from build123d import *

# Parameters (mm, degrees)
SKETCH1_W                                       = 751.2004
SKETCH1_H                                       = 516
SKETCH1_R                                       = 42.5
BOSS_EXTRUDE2_DEPTH                             = 3.175
FILLET1_R                                       = 25
FILLET4_R                                       = 75
SKETCH2_W                                       = 751.2004
SKETCH2_H                                       = 258
CUT_EXTRUDE1_DEPTH                              = 10
FILLET6_R                                       = 10
FILLET7_R                                       = 30
CSK_FOR_10_FLAT_HEAD_MACHINE_SCREW1_D           = 5.1054
CSK_FOR_10_FLAT_HEAD_MACHINE_SCREW1_CSINK_D     = 9.779
CSK_FOR_10_FLAT_HEAD_MACHINE_SCREW1_CSINK_ANGLE = 82
F_1_2_0_5_DIAMETER_HOLE1_D                      = 12.7
F_1_2_0_5_DIAMETER_HOLE1_DEPTH                  = 129.53
F_1_2_0_5_DIAMETER_HOLE1_TIP                    = 3.815464931
CSK_FOR_M4_FLAT_HEAD_MACHINE_SCREW1_D           = 4.5
CSK_FOR_M4_FLAT_HEAD_MACHINE_SCREW1_CSINK_D     = 9.4
CSK_FOR_M4_FLAT_HEAD_MACHINE_SCREW1_CSINK_ANGLE = 90
CIRPATTERN1_COUNT                               = 24
M4_CLEARANCE_HOLE1_D                            = 4.5
SKETCH12_W                                      = 751.2004
SKETCH12_H                                      = 1
CUT_EXTRUDE2_DEPTH                              = 7.35
FILLET8_R                                       = 3.175
FILLET9_R                                       = 5.5
F_3_8_0_375_DIAMETER_HOLE1_TO_CLEAR_4_MM_D      = 9.525
SKETCH18_R                                      = 53
CUT_EXTRUDE3_DEPTH                              = 7.35
F_4_40_TAPPED_HOLE1_D                           = 2.2606
F_4_40_TAPPED_HOLE1_DEPTH                       = 9.53
F_4_40_TAPPED_HOLE1_TIP                         = 0.679152758
FILLET10_R                                      = 0.5


with BuildPart() as part:
    # Sketch1 → Boss-Extrude2 (new body, symmetric)
    with BuildSketch(Plane.XY):
        Rectangle(SKETCH1_W, SKETCH1_H)
        Circle(SKETCH1_R, mode=Mode.SUBTRACT)
        with BuildLine():
            Line((25, 213.516394277), (25, 85))
            Line((25, 85), (-43, 85))
            Line((-43, 85), (-43, 25.710114741))
            ThreePointArc((-43, 25.710114741), (-50.091092447, -0.94469967), (-42, -27.31318363))
            Line((-42, -27.31318363), (-42, -210.832280794))
            ThreePointArc((-42, -210.832280794), (-212.344530207, 33.526871555), (25, 213.516394277))
        make_face(mode=Mode.SUBTRACT)
        with BuildLine():
            Line((-25, -63), (-25, -213.516394277))
            ThreePointArc((-25, -213.516394277), (212.344530207, -33.526871555), (42, 210.832280794))
            Line((42, 210.832280794), (42, 27.31318363))
            ThreePointArc((42, 27.31318363), (47.61154138, -15.593303928), (17.70508892, -46.867257508))
            Line((17.70508892, -46.867257508), (-25, -63))
        make_face(mode=Mode.SUBTRACT)
    extrude(amount=BOSS_EXTRUDE2_DEPTH, both=True)

    # Fillet1
    fillet1_edges = [part.edges().sort_by_distance(p)[0] for p in [
        (42, 27.31318363, 0),
        (-25, -63, 0),
        (-42, -27.31318363, 0),
    ]]
    fillet(fillet1_edges, radius=FILLET1_R)

    # Fillet4
    fillet4_edges = [part.edges().sort_by_distance(p)[0] for p in [
        (42, 210.832280794, 0),
        (-42, -210.832280794, 0),
    ]]
    fillet(fillet4_edges, radius=FILLET4_R)

    # Sketch2 → Cut-Extrude1 (cut)
    with BuildSketch(Plane(origin=(0, 0, -3.175), x_dir=(-1, 0, 0), z_dir=(0, 0, -1))):
        with Locations((0, -129)):
            Rectangle(SKETCH2_W, SKETCH2_H)
    extrude(amount=-CUT_EXTRUDE1_DEPTH, mode=Mode.SUBTRACT)

    # Fillet6
    fillet6_edges = [part.edges().sort_by_distance(p)[0] for p in [
        (-43, 25.710114741, 0),
        (25, 85, 0),
    ]]
    fillet(fillet6_edges, radius=FILLET6_R)

    # Fillet7
    fillet7_edges = [part.edges().sort_by_distance(p)[0] for p in [
        (-43, 85, 0),
    ]]
    fillet(fillet7_edges, radius=FILLET7_R)

    # CSK for #10 Flat Head Machine Screw1 (through all)
    with Locations(Plane(origin=(0, 0, -3.175), x_dir=(-1, 0, 0), z_dir=(0, 0, -1))):
        with Locations((350, 235.5), (350, 250.5), (60, 235.5), (60, 250.5), (-60, 235.5), (-60, 250.5), (-350, 235.5), (-350, 250.5), (310, 235.5), (310, 250.5), (260, 235.5), (260, 250.5), (-310, 235.5), (-310, 250.5), (-260, 235.5), (-260, 250.5), (224, 243), (192, 243), (-224, 243), (-192, 243)):
            CounterSinkHole(CSK_FOR_10_FLAT_HEAD_MACHINE_SCREW1_D / 2, CSK_FOR_10_FLAT_HEAD_MACHINE_SCREW1_CSINK_D / 2, counter_sink_angle=CSK_FOR_10_FLAT_HEAD_MACHINE_SCREW1_CSINK_ANGLE)

    # 1/2 (0.5) Diameter Hole1
    with Locations(Plane(origin=(0, 0, -3.175), x_dir=(-1, 0, 0), z_dir=(0, 0, -1))):
        with Locations((208, 243), (-208, 243)):
            Hole(F_1_2_0_5_DIAMETER_HOLE1_D / 2, depth=F_1_2_0_5_DIAMETER_HOLE1_DEPTH)
            with Locations((0, 0, -(F_1_2_0_5_DIAMETER_HOLE1_DEPTH + F_1_2_0_5_DIAMETER_HOLE1_TIP / 2))):  # 118° drill point
                Cone(0, F_1_2_0_5_DIAMETER_HOLE1_D / 2, F_1_2_0_5_DIAMETER_HOLE1_TIP, mode=Mode.SUBTRACT)

    # CSK for M4 Flat Head Machine Screw1 (through all)
    with Locations(Plane(origin=(0, 0, -3.175), x_dir=(-1, 0, 0), z_dir=(0, 0, -1))):
        with Locations((0, 222)):
            csk_for_m4_flat_head_machine_screw1 = CounterSinkHole(CSK_FOR_M4_FLAT_HEAD_MACHINE_SCREW1_D / 2, CSK_FOR_M4_FLAT_HEAD_MACHINE_SCREW1_CSINK_D / 2, counter_sink_angle=CSK_FOR_M4_FLAT_HEAD_MACHINE_SCREW1_CSINK_ANGLE)

    # CirPattern1: CSK for M4 Flat Head Machine Screw1 ×24 about axis, 13 skipped
    cirpattern1_axis = Axis((0, 0, 0), (0, 0, 1))
    add([csk_for_m4_flat_head_machine_screw1.rotate(cirpattern1_axis, i * 360 / CIRPATTERN1_COUNT) for i in range(1, CIRPATTERN1_COUNT) if i not in (6, 7, 8, 9, 10, 11, 12, 13, 14, 15, 16, 17, 18)], mode=Mode.SUBTRACT)

    # M4 Clearance Hole1 (through all)
    with Locations(Plane(origin=(0, 0, -3.175), x_dir=(-1, 0, 0), z_dir=(0, 0, -1))):
        with Locations((-222, 0), (222, 0)):
            Hole(M4_CLEARANCE_HOLE1_D / 2)

    # Sketch12 → Cut-Extrude2 (cut, through all)
    with BuildSketch(Plane(origin=(0, 0, -3.175), x_dir=(-1, 0, 0), z_dir=(0, 0, -1))):
        Rectangle(SKETCH12_W, SKETCH12_H)
    extrude(amount=-CUT_EXTRUDE2_DEPTH, mode=Mode.SUBTRACT)

    # Fillet8
    fillet8_edges = [part.edges().sort_by_distance(p)[0] for p in [
        (25, 213.516394277, 0),
    ]]
    fillet(fillet8_edges, radius=FILLET8_R)

    # Fillet9
    fillet9_edges = [part.edges().sort_by_distance(p)[0] for p in [
        (-375.6002, 258, 0),
        (375.6002, 258, 0),
    ]]
    fillet(fillet9_edges, radius=FILLET9_R)

    # 3/8 (0.375) Diameter Hole1 to clear  4 mm cap screw (through all)
    with Locations(Plane(origin=(0, 0, -3.175), x_dir=(-1, 0, 0), z_dir=(0, 0, -1))):
        with Locations((-156.977705423, 156.977705423), (156.977705423, 156.977705423)):
            Hole(F_3_8_0_375_DIAMETER_HOLE1_TO_CLEAR_4_MM_D / 2)

    # Sketch18 → Cut-Extrude3 (cut, through all)
    with BuildSketch(Plane(origin=(0, 0, -3.175), x_dir=(-1, 0, 0), z_dir=(0, 0, -1))):
        Circle(SKETCH18_R)
    extrude(amount=-CUT_EXTRUDE3_DEPTH, mode=Mode.SUBTRACT)

    # #4-40 Tapped Hole1
    with Locations(Plane(origin=(0, 0, -3.175), x_dir=(-1, 0, 0), z_dir=(0, 0, -1))):
        with Locations((-30, 51.961524227), (30, 51.961524227)):
            Hole(F_4_40_TAPPED_HOLE1_D / 2, depth=F_4_40_TAPPED_HOLE1_DEPTH)
            with Locations((0, 0, -(F_4_40_TAPPED_HOLE1_DEPTH + F_4_40_TAPPED_HOLE1_TIP / 2))):  # 118° drill point
                Cone(0, F_4_40_TAPPED_HOLE1_D / 2, F_4_40_TAPPED_HOLE1_TIP, mode=Mode.SUBTRACT)

    # Fillet10
    fillet10_edges = [part.edges().sort_by_distance(p)[0] for p in [
        (42.05604293, 32.253515359, 0),
        (-43, 30.98386677, 0),
    ]]
    fillet(fillet10_edges, radius=FILLET10_R)


solid = part.part
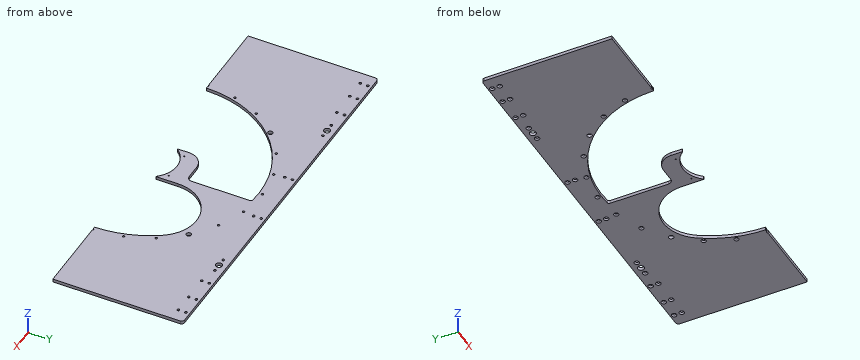
The model under review builds one solid part; all positions refer to its coordinate system, in mm. Give positions to 0.01 mm unless a question says otherwise; leave off trailing zeros. Order: outer loops, then holes, each group sorted by start corner. A loop starts at its lowest first (then second) coordinate and runs counter-clockwise, first axis right, second up. Notation, with made-up numbers: M 41,80 L 88,80 A16 cw 88,105 Z; hole C 42,-21.5 d11. An arc over 180 degrees is marked long. One line per question, with ' | ' between items. Start each with the question number.
1) Wall thickness on L1, parallel to X at y = 157, z = 0.75; L2, parallel to X at y = 98, z = 1.5; L3, parallel to Y at x = 192, z = 0.65: over which ranges is each line inside the solid? List them lowest first. Write a range as from..to.
2) Clearance check with flat-ended pins moving along their axes: P1, Ø6.5, axis at x = 60, y = 250.5, coming from the +Z side (3 decimals); P2, Ø6, axis at x = -310, y = 235.5, coming from the -Z side. State where each tip first meets the part, or that it passes through.
3) Consider section C-C, the plane x = -125. Give the boundary of the cut face in (y, z) (3 decimals), then the cut area to 3 significant figures.
4) Consider section B-B, the plane x = 81. Give the boundary of the cut face in (y, z) (3 decimals), then the cut area to 3 significant figures.
5) Consider section A-A, the plane z = 1. State how many separate pieces and enclosed holes the cut face has, then the cut area to 3 significant figures.
Found:
1) L1: x = -375.6..-161.74, -152.22..-146.85, 25..152.22, 161.74..375.6 | L2: x = -375.6..-191.34, 25..45.05, 191.34..375.6 | L3: y = 96.7..108.76, 113.24..240.45, 245.55..258
2) P1: stops at z = 3.175 | P2: stops at z = -1
3) outline: M 174.898,-3.175 L 258,-3.175 L 258,3.175 L 174.898,3.175 Z | area: 528 mm²
4) outline: M 142.633,-3.175 L 258,-3.175 L 258,3.175 L 142.633,3.175 Z | area: 733 mm²
5) separate pieces: 1 | enclosed holes: 35 | area: 131,000 mm²
